from build123d import *

# Parameters (mm, degrees)
EXTRUDE_1_DEPTH          = 3
PATTERN_CIRCULAR_1_COUNT = 11


with BuildPart() as part:
    # Эскиз2 → Бобышка-Вытянуть1 (new body)
    with BuildSketch(Plane.XY):
        with BuildLine():
            Line((0, 0), (0, 11.712862132))
            ThreePointArc((0, 11.712862132), (1.489205001, 12.208517148), (2.384340039, 13.497756728))
            ThreePointArc((2.384340039, 13.497756728), (3.025331037, 14.908293504), (4.033365809, 16.084877268))
            ThreePointArc((4.033365809, 16.084877268), (4.671932148, 15.911139698), (5.303057959, 15.712062015))
            ThreePointArc((5.303057959, 15.712062015), (5.514961564, 14.177272024), (5.291603749, 12.644107081))
            ThreePointArc((5.291603749, 12.644107081), (5.347623722, 11.075583191), (6.332451358, 9.853486648))
            Line((6.332451358, 9.853486648), (0, 0))
        make_face()
    extrude_1 = extrude(amount=EXTRUDE_1_DEPTH)

    # Круговой массив1: Бобышка-Вытянуть1 ×11 about axis
    pattern_circular_1_axis = Axis((0, 0, 0), (0, 0, 1))
    for i in range(1, PATTERN_CIRCULAR_1_COUNT):
        add(extrude_1.rotate(pattern_circular_1_axis, i * 360 / PATTERN_CIRCULAR_1_COUNT))


solid = part.part
CAD build for the part. Positions are in the model's coordinates, mm. A direction names the side the tool comes from. Coordinates: 2 decimals unless noted, no trailing zeros. Loops run counter-clockwise (first coordinate to the right, second up) from the corner with the lowest first, then second, coordinate; pieces in that order, holes last. Notation, with made-up numbers: (38, 32.25) - (93, 32.25) arc R11 cw to (93, 51.25) - close; hole circle Ø8 at (4, 19.5). An arc over 180 degrees is marked (long way). Write item = value, one per line. Start each with the question number.
Q1. Cut at C-C, the plane y = 4. List the corners of the cut face in (x, z), then the cut area to 3 significant figures.
Q2. Cut at B-B, the plane y = -8.5. List the corners of the cut face in (x, z).
Q3. Which spindle directions (+Z, -Z, +X, -X, +Y, -Y) get a long thin tool onto all of the face, cutting with end or side? Do faces 1 (the cylindrical face through (-8.958, -13.955, 1.479)), 2 (the cylindrical face through (-1.29, -15.18, 1.48)), 3 (the cylindrical face through (9.28, -12.03, 1.48)), 4 (the cylindrical face through (-14.34, -5.13, 1.48)), 5 (the cylindrical face through (10.59, 10.9, 1.48)). Say none if no direction does.
Q4. Flat gauge pins, fed straight in: pin 1 Ø1.5 at (x, z) = (0, 2) entering from +Y; pin 2 Ø1 at (x, z) = (5.5, 1) entering from -Y. Where does each tip first touch, or does it go through?
Q5. Pull direction Y, two halves, no side cores. Call faces 6 (the cylindrical face through (-5.515, 14.156, 1.479)), 7 (the cylindrical face through (-7.09, -13.44, 1.48)), 8 (the cylindrical face through (4.663, 15.914, 1.479)): pulls with the +Y half, pulls with the -Y half, needs draft (parallel to the pull), parting line crosses it, or undercut.
Q6. Drill centre lines: L1, parallel to X at y = -12.5, z = 2.6; L2, parallel to X at y = 3, z = 0.65; L3, parallel to X at y = -13.5, z = 1.2. Where is each one in solid material? Low to high.
Q7. Cut at A-A, the plane y = -13. List the corners of the cut face in (x, z), then the cut area to 3 significant figures.
Computed:
q1.outline = (-11.31, 0) - (11.31, 0) - (11.31, 3) - (-11.31, 3) - close
q1.area = 67.9 mm²
q2.outline = (-8.38, 0) - (8.38, 0) - (8.38, 3) - (-8.38, 3) - close
q3.face_1 = +Z, -Z, -X, -Y
q3.face_2 = +Z, -Z, -Y
q3.face_3 = +Z, -Z, +X
q3.face_4 = +Z, -Z, -X
q3.face_5 = +Z, -Z, +Y
q4.pin_1 = 11.83
q4.pin_2 = -12.15
q5.face_6 = undercut
q5.face_7 = pulls with the -Y half
q5.face_8 = pulls with the +Y half
q6.L1 = -9.4 to -6.24, -1.78 to 1.78, 6.24 to 9.4
q6.L2 = -16.31 to 16.31
q6.L3 = -9.51 to -7.16, -1.52 to 1.52, 7.16 to 9.51
q7.outline = (-9.48, 0) - (-6.64, 0) - (-6.64, 3) - (-9.48, 3) - close; (-1.59, 0) - (1.59, 0) - (1.59, 3) - (-1.59, 3) - close; (6.64, 0) - (9.48, 0) - (9.48, 3) - (6.64, 3) - close
q7.area = 26.6 mm²
